Geometry check sheet. Reference: drawing and pictorial views, mm from the part's lowest x, y, z. A direction names the side the tool comes from. Coordinates: 2 decimals unless noted, no trailing zeros. Loops run counter-clockwise (first coordinate to the right, second up) from the corner with the lowest first, then second, coordinate; pieces in that order, holes last. Notation, with made-up numbers: (-11, 76) -> (41, 76) arc R35 cw to (41, 108) -> close; hole circle Ø10 at (3, 26.25). An arc over 180 degrees is marked (long way). Use one line per item in the form item = value.
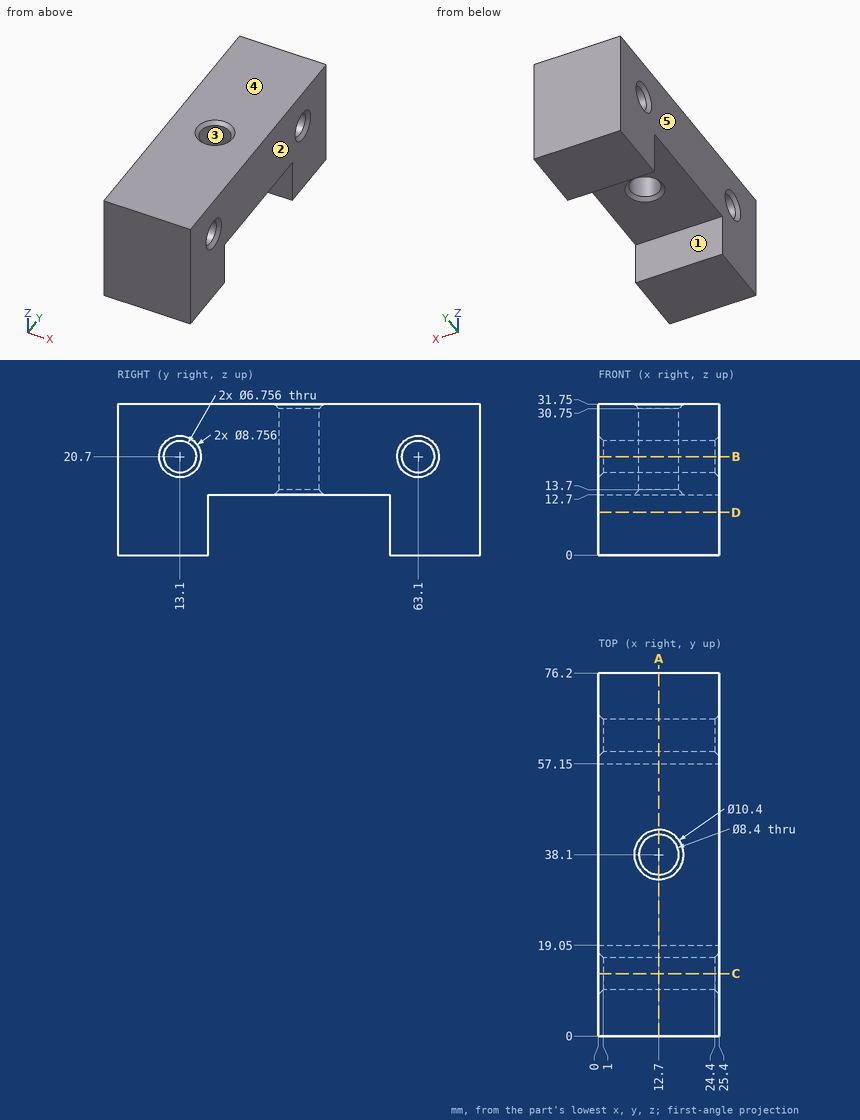
(1) Go/stop test with flat-tipped pins: P1, Ø12.5, axis at x = 12.5, y = 44.5, coming from the -Z side; P2, Ø8, axis at y = 63.1, z = 20.7, coming from the -X side. Record where each tip stops, or that it passes through.
Established:
P1 = 12.7
P2 = 0.38
(2) Section check B-B, the plane z = 20.7. Record the boundary of the cut face in (x, y), plus the area to 3 significant figures.
Established:
outline = (0, 0) -> (25.4, 0) -> (25.4, 8.72) -> (24.4, 9.72) -> (1, 9.72) -> (0, 8.72) -> close; (0, 17.48) -> (1, 16.48) -> (24.4, 16.48) -> (25.4, 17.48) -> (25.4, 58.72) -> (24.4, 59.72) -> (1, 59.72) -> (0, 58.72) -> close; (0, 67.48) -> (1, 66.48) -> (24.4, 66.48) -> (25.4, 67.48) -> (25.4, 76.2) -> (0, 76.2) -> close; hole circle Ø8.4 at (12.7, 38.1)
area = 1,530 mm²
(3) Section check C-C, the plane y = 13.1. Record the boundary of the cut face in (x, z), plus the area to 3 significant figures.
Established:
outline = (0, 0) -> (25.4, 0) -> (25.4, 16.32) -> (24.4, 17.32) -> (1, 17.32) -> (0, 16.32) -> close; (0, 25.08) -> (1, 24.08) -> (24.4, 24.08) -> (25.4, 25.08) -> (25.4, 31.75) -> (0, 31.75) -> close
area = 633 mm²
(4) Mould release check, pull along X, two halves, no side actions. Record for the marked faces 3, 4 and 5: +X half, -X half, draft (parallel to the pull), parting line (faces both ways), or undercut.
Established:
face_3 = undercut
face_4 = draft
face_5 = -X half
(5) Tool access check on the marked faces 1 and 2. Record the directions out of +Z, -Z, +X, -X, +Y, -Y that give a thin tool (end or side, any length) a straight path to the whole face; none if there is none.
Established:
face_1 = -Z, +X, -X
face_2 = +Z, -Z, +X, +Y, -Y
(6) Section check A-A, the plane x = 12.7. Record the boundary of the cut face in (y, z), plus the area to 3 significant figures.
Established:
outline = (0, 0) -> (19.05, 0) -> (19.05, 12.7) -> (32.9, 12.7) -> (33.9, 13.7) -> (33.9, 30.75) -> (32.9, 31.75) -> (0, 31.75) -> close; (42.3, 13.7) -> (43.3, 12.7) -> (57.15, 12.7) -> (57.15, 0) -> (76.2, 0) -> (76.2, 31.75) -> (43.3, 31.75) -> (42.3, 30.75) -> close; hole circle Ø6.76 at (13.1, 20.7); hole circle Ø6.76 at (63.1, 20.7)
area = 1,700 mm²
(7) Scan lines: line 1 along Z through (x, y) = (5.75, 63.1); line 2 along Y through (x, z) = (9.5, 12.5); line 3 along Y through (x, z) = (23.75, 23) (1 decimal). Record each from-to range of solid material in increasing order.
Established:
line_1 = 0 to 17.32, 24.08 to 31.75
line_2 = 0 to 19.05, 57.15 to 76.2
line_3 = 0 to 10.6, 15.6 to 60.6, 65.6 to 76.2
(8) Section check D-D, the plane z = 9. Record the boundary of the cut face in (x, y), plus the area to 3 significant figures.
Established:
outline = (0, 0) -> (25.4, 0) -> (25.4, 19.05) -> (0, 19.05) -> close; (0, 57.15) -> (25.4, 57.15) -> (25.4, 76.2) -> (0, 76.2) -> close
area = 968 mm²
